Geometry: final body of the model. Coordinates: model frame, mm. Give positions to 0.01 mm unless a question says otherwise; leave off trailing zeros. Order: outer loops, then holes, each group sorted by start corner. A loop starts at its lowest first (then second) coordinate and runs counter-clockwise, first axis right, second up. Notation, with made-up numbers: (15, -33) - (60, -33) arc R20 cw to (60, 5) - close; hole circle Ø9 at (21.25, 63). An arc over 180 degrees is marked (long way). Put each result on its own line as item: value. Start each with the question number.
1. First-contact query: P1, Ø3, axis at y = -3.5, z = 10, coming from the +X side (3 decimals); P2, Ø1.9, axis at y = -4.5, z = -11, coming from the -X side (3 decimals). Flat tips, straight axial feed; report the tip coordinate or a pass-through.
2. Section A-A on x = 75. Return the cut outline in (y, z), plus the area to 3 significant figures.
3. Section B-B on z = -16.5. Count the separate pieces of the cut face and the enclosed holes in it, plus the area to 3 significant figures.
4. Ray query, line 1 along Z through (x, y) = (119.5, -5.25). Return the intervals inside material, ascending. Write a range as from..to.
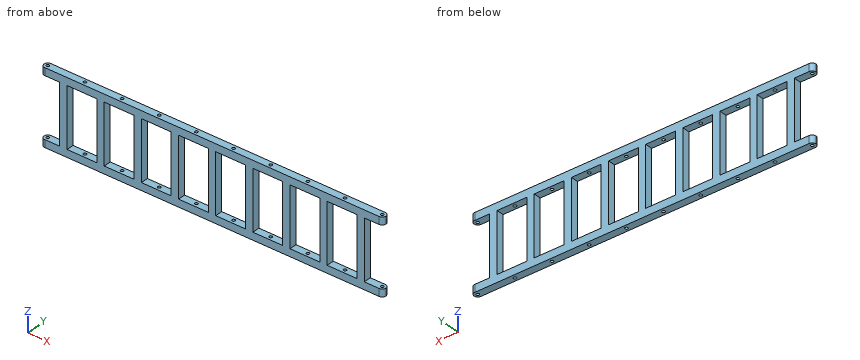
from build123d import *

# Parameters (mm, degrees)
SKETCH1_W           = 25.4
SKETCH1_H           = 50.8
BOSS_EXTRUDE1_DEPTH = 6.35
CUT_EXTRUDE1_REACH  = 161.384
SKETCH2_R           = 1.27
FILLET2_R           = 3.175


with BuildPart() as part:
    # Sketch1 → Boss-Extrude1 (new body)
    with BuildSketch(Plane(origin=(0, 0, 0), x_dir=(1, 0, 0), z_dir=(0, 1, 0))):
        Polygon((-146.05, 25.4), (-130.175, 25.4), (-130.175, -25.4), (-146.05, -25.4), (-146.05, -31.75), (146.05, -31.75), (146.05, -25.4), (130.175, -25.4), (130.175, 25.4), (146.05, 25.4), (146.05, 31.75), (-146.05, 31.75), align=None)
        with Locations((-15.875, 0)):
            Rectangle(SKETCH1_W, SKETCH1_H, mode=Mode.SUBTRACT)
        with Locations((111.125, 0)):
            Rectangle(SKETCH1_W, SKETCH1_H, mode=Mode.SUBTRACT)
        with Locations((-47.625, 0)):
            Rectangle(SKETCH1_W, SKETCH1_H, mode=Mode.SUBTRACT)
        with Locations((-79.375, 0)):
            Rectangle(SKETCH1_W, SKETCH1_H, mode=Mode.SUBTRACT)
        with Locations((-111.125, 0)):
            Rectangle(SKETCH1_W, SKETCH1_H, mode=Mode.SUBTRACT)
        with Locations((79.375, 0)):
            Rectangle(SKETCH1_W, SKETCH1_H, mode=Mode.SUBTRACT)
        with Locations((47.625, 0)):
            Rectangle(SKETCH1_W, SKETCH1_H, mode=Mode.SUBTRACT)
        with Locations((15.875, 0)):
            Rectangle(SKETCH1_W, SKETCH1_H, mode=Mode.SUBTRACT)
    extrude(amount=-BOSS_EXTRUDE1_DEPTH)

    # Cut-Extrude1: up to this face of the body (flat: up to its plane)
    cut_extrude1_end = Plane(part.part.faces().sort_by_distance((0, -3.175, -31.75))[0])
    # Sketch2 → Cut-Extrude1 (cut, up to the picked face)
    with BuildSketch(Plane.XY.offset(31.75), mode=Mode.PRIVATE) as cut_extrude1_sk1:
        with Locations((-142.875, -3.175)):
            Circle(SKETCH2_R)
    cut_extrude1_tool1 = split(extrude(cut_extrude1_sk1.sketch, amount=-CUT_EXTRUDE1_REACH, mode=Mode.PRIVATE), bisect_by=cut_extrude1_end, keep=Keep.BOTH, mode=Mode.PRIVATE)
    # Sketch2 → Cut-Extrude1 (cut, up to the picked face)
    with BuildSketch(Plane.XY.offset(31.75), mode=Mode.PRIVATE) as cut_extrude1_sk2:
        with Locations((-111.125, -3.175)):
            Circle(SKETCH2_R)
    cut_extrude1_tool2 = split(extrude(cut_extrude1_sk2.sketch, amount=-CUT_EXTRUDE1_REACH, mode=Mode.PRIVATE), bisect_by=cut_extrude1_end, keep=Keep.BOTH, mode=Mode.PRIVATE)
    # Sketch2 → Cut-Extrude1 (cut, up to the picked face)
    with BuildSketch(Plane.XY.offset(31.75), mode=Mode.PRIVATE) as cut_extrude1_sk3:
        with Locations((-79.375, -3.175)):
            Circle(SKETCH2_R)
    cut_extrude1_tool3 = split(extrude(cut_extrude1_sk3.sketch, amount=-CUT_EXTRUDE1_REACH, mode=Mode.PRIVATE), bisect_by=cut_extrude1_end, keep=Keep.BOTH, mode=Mode.PRIVATE)
    # Sketch2 → Cut-Extrude1 (cut, up to the picked face)
    with BuildSketch(Plane.XY.offset(31.75), mode=Mode.PRIVATE) as cut_extrude1_sk4:
        with Locations((-47.625, -3.175)):
            Circle(SKETCH2_R)
    cut_extrude1_tool4 = split(extrude(cut_extrude1_sk4.sketch, amount=-CUT_EXTRUDE1_REACH, mode=Mode.PRIVATE), bisect_by=cut_extrude1_end, keep=Keep.BOTH, mode=Mode.PRIVATE)
    # Sketch2 → Cut-Extrude1 (cut, up to the picked face)
    with BuildSketch(Plane.XY.offset(31.75), mode=Mode.PRIVATE) as cut_extrude1_sk5:
        with Locations((-15.875, -3.175)):
            Circle(SKETCH2_R)
    cut_extrude1_tool5 = split(extrude(cut_extrude1_sk5.sketch, amount=-CUT_EXTRUDE1_REACH, mode=Mode.PRIVATE), bisect_by=cut_extrude1_end, keep=Keep.BOTH, mode=Mode.PRIVATE)
    # Sketch2 → Cut-Extrude1 (cut, up to the picked face)
    with BuildSketch(Plane.XY.offset(31.75), mode=Mode.PRIVATE) as cut_extrude1_sk6:
        with Locations((15.875, -3.175)):
            Circle(SKETCH2_R)
    cut_extrude1_tool6 = split(extrude(cut_extrude1_sk6.sketch, amount=-CUT_EXTRUDE1_REACH, mode=Mode.PRIVATE), bisect_by=cut_extrude1_end, keep=Keep.BOTH, mode=Mode.PRIVATE)
    # Sketch2 → Cut-Extrude1 (cut, up to the picked face)
    with BuildSketch(Plane.XY.offset(31.75), mode=Mode.PRIVATE) as cut_extrude1_sk7:
        with Locations((47.625, -3.175)):
            Circle(SKETCH2_R)
    cut_extrude1_tool7 = split(extrude(cut_extrude1_sk7.sketch, amount=-CUT_EXTRUDE1_REACH, mode=Mode.PRIVATE), bisect_by=cut_extrude1_end, keep=Keep.BOTH, mode=Mode.PRIVATE)
    # Sketch2 → Cut-Extrude1 (cut, up to the picked face)
    with BuildSketch(Plane.XY.offset(31.75), mode=Mode.PRIVATE) as cut_extrude1_sk8:
        with Locations((79.375, -3.175)):
            Circle(SKETCH2_R)
    cut_extrude1_tool8 = split(extrude(cut_extrude1_sk8.sketch, amount=-CUT_EXTRUDE1_REACH, mode=Mode.PRIVATE), bisect_by=cut_extrude1_end, keep=Keep.BOTH, mode=Mode.PRIVATE)
    # Sketch2 → Cut-Extrude1 (cut, up to the picked face)
    with BuildSketch(Plane.XY.offset(31.75), mode=Mode.PRIVATE) as cut_extrude1_sk9:
        with Locations((111.125, -3.175)):
            Circle(SKETCH2_R)
    cut_extrude1_tool9 = split(extrude(cut_extrude1_sk9.sketch, amount=-CUT_EXTRUDE1_REACH, mode=Mode.PRIVATE), bisect_by=cut_extrude1_end, keep=Keep.BOTH, mode=Mode.PRIVATE)
    # Sketch2 → Cut-Extrude1 (cut, up to the picked face)
    with BuildSketch(Plane.XY.offset(31.75), mode=Mode.PRIVATE) as cut_extrude1_sk10:
        with Locations((142.875, -3.175)):
            Circle(SKETCH2_R)
    cut_extrude1_tool10 = split(extrude(cut_extrude1_sk10.sketch, amount=-CUT_EXTRUDE1_REACH, mode=Mode.PRIVATE), bisect_by=cut_extrude1_end, keep=Keep.BOTH, mode=Mode.PRIVATE)
    add(cut_extrude1_tool1.solids().sort_by(Axis((-142.875, -3.175, 31.75), (0, 0, -1)))[0], mode=Mode.SUBTRACT)
    add(cut_extrude1_tool2.solids().sort_by(Axis((-111.125, -3.175, 31.75), (0, 0, -1)))[0], mode=Mode.SUBTRACT)
    add(cut_extrude1_tool3.solids().sort_by(Axis((-79.375, -3.175, 31.75), (0, 0, -1)))[0], mode=Mode.SUBTRACT)
    add(cut_extrude1_tool4.solids().sort_by(Axis((-47.625, -3.175, 31.75), (0, 0, -1)))[0], mode=Mode.SUBTRACT)
    add(cut_extrude1_tool5.solids().sort_by(Axis((-15.875, -3.175, 31.75), (0, 0, -1)))[0], mode=Mode.SUBTRACT)
    add(cut_extrude1_tool6.solids().sort_by(Axis((15.875, -3.175, 31.75), (0, 0, -1)))[0], mode=Mode.SUBTRACT)
    add(cut_extrude1_tool7.solids().sort_by(Axis((47.625, -3.175, 31.75), (0, 0, -1)))[0], mode=Mode.SUBTRACT)
    add(cut_extrude1_tool8.solids().sort_by(Axis((79.375, -3.175, 31.75), (0, 0, -1)))[0], mode=Mode.SUBTRACT)
    add(cut_extrude1_tool9.solids().sort_by(Axis((111.125, -3.175, 31.75), (0, 0, -1)))[0], mode=Mode.SUBTRACT)
    add(cut_extrude1_tool10.solids().sort_by(Axis((142.875, -3.175, 31.75), (0, 0, -1)))[0], mode=Mode.SUBTRACT)

    # Fillet2
    fillet2_edges = [part.edges().sort_by_distance(p)[0] for p in [
        (-146.05, -6.35, 28.575),
        (-146.05, 0, 28.575),
        (-146.05, -6.35, -28.575),
        (-146.05, 0, -28.575),
        (146.05, -6.35, -28.575),
        (146.05, 0, -28.575),
        (146.05, -6.35, 28.575),
        (146.05, 0, 28.575),
    ]]
    fillet(fillet2_edges, radius=FILLET2_R - 0.0001)  # a hair under: the kernel refuses the full size


solid = part.part
Resolved:
1. P1: x = 130.175
1. P2: x = -130.175
2. outline: (-6.35, -31.75) - (0, -31.75) - (0, -25.4) - (-6.35, -25.4) - close; (-6.35, 25.4) - (0, 25.4) - (0, 31.75) - (-6.35, 31.75) - close
2. area: 80.6 mm^2
3. separate pieces: 9
3. enclosed holes: 0
3. area: 363 mm^2
4. line 1: -31.75..-25.4, 25.4..31.75
